Model file for the job. Use its own axes, mm. Give positions to 0.01 mm unless a question says otherwise; leave off trailing zeros. Loops run counter-clockwise (first coordinate to the right, second up) from the corner with the lowest first, then second, coordinate; pieces in that order, holes last. Notation, with made-up numbers: M 13,72 L 46,72 A18 ccw 46,102 Z; hole C -30,-18.75 d7. An arc over 180 degrees is marked long. Answer in a Markdown table with one row per item.
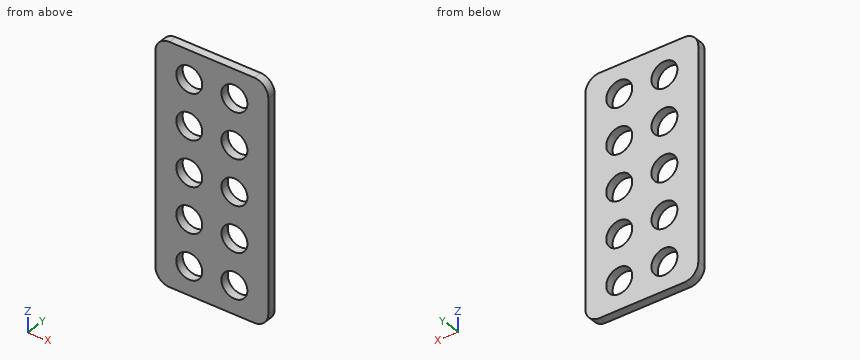
```python
from build123d import *

# Parameters (mm, degrees)
F0_W     = 20
F0_H     = 84
F0_R     = 4.6
F1_DEPTH = 3
F2_R     = 5


with BuildPart() as f1:
    # F0 (on Front) → F1 (new body)
    with BuildSketch(Plane.XZ):
        with Locations((-33.898029, 2.626098)):
            Rectangle(F0_W, F0_H)
        with Locations((-31.898029, -29.373902)):
            Circle(F0_R, mode=Mode.SUBTRACT)
        with Locations((-31.898029, -13.373902)):
            Circle(F0_R, mode=Mode.SUBTRACT)
        with Locations((-31.898029, 2.626098)):
            Circle(F0_R, mode=Mode.SUBTRACT)
        with Locations((-31.898029, 18.626098)):
            Circle(F0_R, mode=Mode.SUBTRACT)
        with Locations((-31.898029, 34.626098)):
            Circle(F0_R, mode=Mode.SUBTRACT)
        with Locations((-13.898029, 2.626098)):
            Rectangle(F0_W, F0_H)
        with Locations((-15.898029, -29.373902)):
            Circle(F0_R, mode=Mode.SUBTRACT)
        with Locations((-15.898029, -13.373902)):
            Circle(F0_R, mode=Mode.SUBTRACT)
        with Locations((-15.898029, 2.626098)):
            Circle(F0_R, mode=Mode.SUBTRACT)
        with Locations((-15.898029, 18.626098)):
            Circle(F0_R, mode=Mode.SUBTRACT)
        with Locations((-15.898029, 34.626098)):
            Circle(F0_R, mode=Mode.SUBTRACT)
    extrude(amount=F1_DEPTH)

    # F2
    f2_edges = [f1.edges().sort_by_distance(p)[0] for p in [
        (-43.898029, -1.5, 44.626098),
        (-3.898029, -1.5, 44.626098),
        (-3.898029, -1.5, -39.373902),
        (-43.898029, -1.5, -39.373902),
    ]]
    fillet(f2_edges, radius=F2_R)


solid = f1.part
```
(1) Wall check: L1, parallel to X at y = -1.95, z = 18.5; L2, parallel to X at y = -2.25, z = 36; L3, parallel to Z at x = -13, y = -1.1. Give the ranges that are in metal, low to high.
Established:
| item | result |
|---|---|
| L1 | x = -43.9 to -36.5, -27.3 to -20.5, -11.3 to -3.9 |
| L2 | x = -43.9 to -36.29, -27.51 to -20.29, -11.51 to -3.9 |
| L3 | z = -39.37 to -32.95, -25.8 to -16.95, -9.8 to -0.95, 6.2 to 15.05, 22.2 to 31.05, 38.2 to 44.63 |
(2) Saw through at B-B, the plane y = -1.1. Count the separate pieces of the cut face and the enclosed holes in it, and give its area (3 significant figures).
Established:
| item | result |
|---|---|
| separate pieces | 1 |
| enclosed holes | 10 |
| area | 2,670 mm2 |
(3) Saw through at C-C, the plane x = -33. Give the cut face in (y, z), and give its area (3 significant figures).
Established:
| item | result |
|---|---|
| outline | M -3,-39.37 L 0,-39.37 L 0,-33.84 L -3,-33.84 Z; M -3,-24.91 L 0,-24.91 L 0,-17.84 L -3,-17.84 Z; M -3,-8.91 L 0,-8.91 L 0,-1.84 L -3,-1.84 Z; M -3,7.09 L 0,7.09 L 0,14.16 L -3,14.16 Z; M -3,23.09 L 0,23.09 L 0,30.16 L -3,30.16 Z; M -3,39.09 L 0,39.09 L 0,44.63 L -3,44.63 Z |
| area | 118 mm2 |
(4) Flat gauge pin, fed straight in: P1, Ø7.5, axis at x = -15.9, z = -29.37, coming from the +Y side. Where does the tip first touch, or does it go through?
Established:
| item | result |
|---|---|
| P1 | passes through |
(5) Saw through at A-A, the plane x = -18. Give the cut face in (y, z).
Established:
| item | result |
|---|---|
| outline | M -3,-39.37 L 0,-39.37 L 0,-33.47 L -3,-33.47 Z; M -3,-25.28 L 0,-25.28 L 0,-17.47 L -3,-17.47 Z; M -3,-9.28 L 0,-9.28 L 0,-1.47 L -3,-1.47 Z; M -3,6.72 L 0,6.72 L 0,14.53 L -3,14.53 Z; M -3,22.72 L 0,22.72 L 0,30.53 L -3,30.53 Z; M -3,38.72 L 0,38.72 L 0,44.63 L -3,44.63 Z |
